The listing builds one solid part. Answer for the finished solid, in the listing's coordinates (mm). Face numbers are marked on the shaded views. A direction names the side the tool comes from. Round coordinates to 2 decimals unless told otherwise and drop trailing zeros. Loops run counter-clockwise (first coordinate to the right, second up) from the corner with the lowest first, then second, coordinate; pieces in that order, holes last. Notation, with made-up numbers: (14.5, 14.5) -> (35.5, 14.5) arc R19 cw to (35.5, 39.5) -> close; hole circle Ø6 at (-31.75, 16.5). An arc over 180 degrees is marked (long way). Answer in a Markdown table with one row per item. Add a question column.
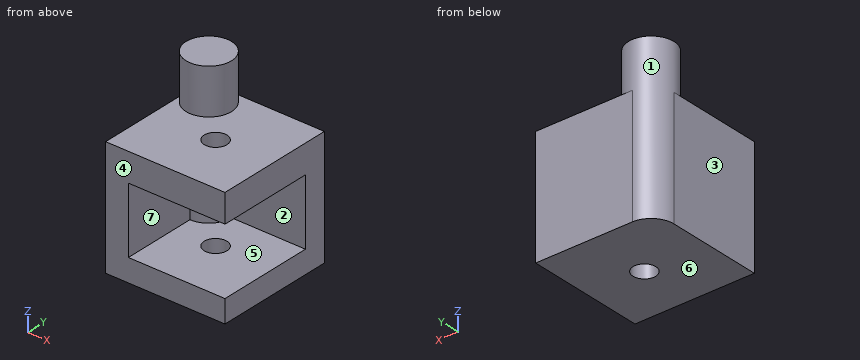
```python
from build123d import *
from build123d.topology import SkipClean

# Parameters (mm, degrees)
BOSS_EXTRUDE1_DEPTH     = 11.7
BOSS_EXTRUDE4_START     = 8
SKETCH1_6_R             = 4
BOSS_EXTRUDE4_DEPTH     = 8
BOSS_EXTRUDE5_START     = -11.7
SKETCH1_7_R             = 2
BOSS_EXTRUDE5_DEPTH     = 4
BOSS_EXTRUDE6_START     = 5
SKETCH1_8_R             = 2
BOSS_EXTRUDE6_DEPTH     = 5
BOSS_EXTRUDE7_START     = 8
BOSS_EXTRUDE7_OUTLINE_R = 4
BOSS_EXTRUDE7_DEPTH     = 5
SKETCH2_W               = 7
SKETCH2_H               = 10
SKETCH2_H_2             = 7
SKETCH2_W_2             = 10
BOSS_EXTRUDE8_DEPTH     = 5
BOSS_EXTRUDE9_START     = -20.7
SKETCH2_3_W             = 7
SKETCH2_3_H             = 10
SKETCH2_3_W_2           = 10
SKETCH2_3_H_2           = 7
BOSS_EXTRUDE9_DEPTH     = 4


# Read off the part's stored shape, not the designer's step: Boss-Extrude7
with BuildPart() as part:
    # Sketch1 → Boss-Extrude1 (new body)
    with BuildSketch(Plane.XY):
        with BuildLine():
            Line((-36, -4), (-29, -4))
            Line((-29, -4), (-29, 0))
            Line((-29, 0), (-46, 0))
            ThreePointArc((-46, 0), (-43.171572875, -1.171572875), (-42, -4))
            Line((-42, -4), (-36, -4))
        make_face()
        with BuildLine():
            ThreePointArc((-46, -8), (-43.171572875, -6.828427125), (-42, -4))
            Line((-42, -4), (-46, -4))
            Line((-46, -4), (-46, -8))
        make_face()
        with BuildLine():
            Line((-46, -4), (-42, -4))
            ThreePointArc((-42, -4), (-43.171572875, -1.171572875), (-46, 0))
            Line((-46, 0), (-46, -4))
        make_face()
        with BuildLine():
            Line((-46, -4), (-46, 0))
            ThreePointArc((-46, 0), (-48.828427125, -1.171572875), (-50, -4))
            Line((-50, -4), (-46, -4))
        make_face()
        with BuildLine():
            Line((-46, -8), (-46, -4))
            Line((-46, -4), (-50, -4))
            ThreePointArc((-50, -4), (-48.828427125, -6.828427125), (-46, -8))
        make_face()
        with BuildLine():
            Line((-46, -14), (-46, -8))
            ThreePointArc((-46, -8), (-48.828427125, -6.828427125), (-50, -4))
            Line((-50, -4), (-50, -21))
            Line((-50, -21), (-46, -21))
            Line((-46, -21), (-46, -14))
        make_face()
    extrude(amount=-BOSS_EXTRUDE1_DEPTH)

    # Sketch1<6> → Boss-Extrude4 (add)
    with BuildSketch(Plane.XY.offset(BOSS_EXTRUDE4_START)):
        with Locations((-46, -4)):
            Circle(SKETCH1_6_R)
    extrude(amount=-BOSS_EXTRUDE4_DEPTH)

    # Sketch1<7> → Boss-Extrude5 (add)
    with SkipClean():  # the faces are left unmerged after this step: merging them gives an invalid solid
        with BuildSketch(Plane.XY.offset(BOSS_EXTRUDE5_START)):
            with BuildLine():
                Line((-36, -4), (-29, -4))
                Line((-29, -4), (-29, 0))
                Line((-29, 0), (-46, 0))
                ThreePointArc((-46, 0), (-48.828427125, -1.171572875), (-50, -4))
                Line((-50, -4), (-50, -21))
                Line((-50, -21), (-46, -21))
                Line((-46, -21), (-46, -14))
                Line((-46, -14), (-36, -14))
                Line((-36, -14), (-36, -4))
            make_face()
            with Locations((-38.878679656, -11.121320344)):
                Circle(SKETCH1_7_R, mode=Mode.SUBTRACT)
        extrude(amount=-BOSS_EXTRUDE5_DEPTH)

    # Sketch1<8> → Boss-Extrude6 (add)
    # profile 1 of 3: a face of its own
    with BuildSketch(Plane.XY.offset(BOSS_EXTRUDE6_START)):
        with BuildLine():
            Line((-46, -14), (-46, -8))
            ThreePointArc((-46, -8), (-48.828427125, -6.828427125), (-50, -4))
            Line((-50, -4), (-50, -21))
            Line((-50, -21), (-46, -21))
            Line((-46, -21), (-46, -14))
        make_face()
    # profile 2 of 3: a face of its own
    with BuildSketch(Plane.XY.offset(BOSS_EXTRUDE6_START)):
        with BuildLine():
            Line((-36, -14), (-36, -4))
            Line((-36, -4), (-42, -4))
            ThreePointArc((-42, -4), (-43.171572875, -6.828427125), (-46, -8))
            Line((-46, -8), (-46, -14))
            Line((-46, -14), (-36, -14))
        make_face()
        with Locations((-38.878679656, -11.121320344)):
            Circle(SKETCH1_8_R, mode=Mode.SUBTRACT)
    # profile 3 of 3: a face of its own
    with BuildSketch(Plane.XY.offset(BOSS_EXTRUDE6_START)):
        with BuildLine():
            Line((-36, -4), (-29, -4))
            Line((-29, -4), (-29, 0))
            Line((-29, 0), (-46, 0))
            ThreePointArc((-46, 0), (-43.171572875, -1.171572875), (-42, -4))
            Line((-42, -4), (-36, -4))
        make_face()
    extrude(amount=-BOSS_EXTRUDE6_DEPTH)

    # Boss-Extrude7 outline → Boss-Extrude7 (add)
    with BuildSketch(Plane.XY.offset(BOSS_EXTRUDE7_START)):
        with Locations((-46, -4)):
            Circle(BOSS_EXTRUDE7_OUTLINE_R)
    extrude(amount=BOSS_EXTRUDE7_DEPTH)

    # Sketch2 → Boss-Extrude8 (add)
    with BuildSketch(Plane.XY.offset(5)):
        with Locations((-32.5, -9)):
            Rectangle(SKETCH2_W, SKETCH2_H)
        with Locations((-32.5, -17.5)):
            Rectangle(SKETCH2_W, SKETCH2_H_2)
        with Locations((-41, -17.5)):
            Rectangle(SKETCH2_W_2, SKETCH2_H_2)
    extrude(amount=-BOSS_EXTRUDE8_DEPTH)

    # Sketch2<3> → Boss-Extrude9 (add)
    with BuildSketch(Plane.XY.offset(5).offset(BOSS_EXTRUDE9_START)):
        with Locations((-32.5, -9)):
            Rectangle(SKETCH2_3_W, SKETCH2_3_H)
        with Locations((-41, -17.5)):
            Rectangle(SKETCH2_3_W_2, SKETCH2_3_H_2)
        with Locations((-32.5, -17.5)):
            Rectangle(SKETCH2_3_W, SKETCH2_3_H_2)
    extrude(amount=BOSS_EXTRUDE9_DEPTH)


solid = part.part
```
Item 1: Section D-D, the plane z = 3.25 is taken. Write down the section's boundary in (x, y).
Item 2: The mould has two halves that part along Z. Classify the marked faces 4, 5, 6 and 7: +Z half, -Z half, draft (parallel to the pull), parting line (faces both ways), or undercut.
Item 3: Flat-ended cylindrical pins translate along their axes: P1, Ø1, axis at y = -5.5, z = -6.5, coming from the +X side; P2, Ø5, axis at x = -40, z = -3, coming from the -Y side; P3, Ø8.5, axis at x = -34.5, y = -14, coming from the +Z side. Find the tip coordinate at first contact, or state that the pin passes through.
Item 4: Consider L1, parallel to Z at x = -43, y = -13.75; L2, parallel to Z at x = -48.25, y = -15.75; L3, parallel to Y at x = -31.25, z = -10. Determine where each line is inside the solid, lowest interval first. Write a range as from..to.
Item 5: For the marked faces 1, 2 and 3, determine the directions among +Z, -Z, +X, -X, +Y, -Y from which every point of the face is accessible in a straight line to the end or side of a thin tool.
Item 6: Section C-C, the plane x = -34 is taken. Write down the section's boundary in (y, z), and give its area (3 significant figures).
Item 7: Section A-A, the plane y = -12.5 is taken. Write down the section's boundary in (x, z).
Item 8: Section B-B, the plane z = -8.5 is taken. Write down the section's boundary in (x, y), and give its area (3 significant figures).
Here are the results:
| question | item | result |
|---|---|---|
| 1 | outline | (-50, -21) -> (-29, -21) -> (-29, 0) -> (-46, 0) arc R4 ccw to (-50, -4) -> close; hole circle Ø4 at (-38.88, -11.12) |
| 2 | face 4 | draft |
| 2 | face 5 | undercut |
| 2 | face 6 | -Z half |
| 2 | face 7 | undercut |
| 3 | P1 | stops at x = -42.13 |
| 3 | P2 | stops at y = -5.94 |
| 3 | P3 | stops at z = 5 |
| 4 | L1 | z = -15.7..-11.7, 0..5 |
| 4 | L2 | z = -15.7..5 |
| 4 | L3 | y = -4..0 |
| 5 | face 1 | +Z |
| 5 | face 2 | +X, -Y |
| 5 | face 3 | +Z, -Z, -X, +Y, -Y |
| 6 | outline | (-21, -15.7) -> (0, -15.7) -> (0, 5) -> (-21, 5) -> (-21, 0) -> (-4, 0) -> (-4, -11.7) -> (-21, -11.7) -> close |
| 6 | area | 236 mm² |
| 7 | outline | (-50, -15.7) -> (-40.33, -15.7) -> (-40.33, -11.7) -> (-46, -11.7) -> (-46, 0) -> (-40.33, 0) -> (-40.33, 5) -> (-50, 5) -> close; (-37.43, -15.7) -> (-29, -15.7) -> (-29, -11.7) -> (-37.43, -11.7) -> close; (-37.43, 0) -> (-29, 0) -> (-29, 5) -> (-37.43, 5) -> close |
| 8 | outline | (-50, -21) -> (-46, -21) -> (-46, -8) arc R4 ccw to (-42, -4) -> (-29, -4) -> (-29, 0) -> (-46, 0) arc R4 ccw to (-50, -4) -> close |
| 8 | area | 161 mm² |
